Check sheet for the modelled part. Datum: model origin and axes. Units: mm. A direction names the side the tool comes from. Round coordinates to 2 decimals unless told otherwise and drop trailing zeros. Order: outer loops, then holes, each group sorted by start corner. A loop starts at its lowest first (then second) coordinate and runs counter-clockwise, first axis right, second up. Notation, with made-up numbers: M 85.25,33 L 112.25,33 A9 cw 112.25,40 Z; hole C -38.75,-36 d3. An arc over 180 degrees is marked long. One line per item, written item: value. Start each with the question number.
(1) Depth check by flat-ended pin: pin 1 Ø6 at (x, y) = (2, -2) entering from +Z. Enter the tip coordinate at first touch or a pass-through.
(2) Release check for a two-part mould opening along Z. For faces 1 (the face through (0, -11, 3)), 2 (the face through (-1, -1, 0)), 3 (the face through (-10.5, -1, 9)) record: released by +Z, released by -Z, zero draft, split by the parting line, or undercut.
(3) Cross-section at D-D, the plane x = 2. Enter the section's corners in (y, z).
(4) Cross-section at C-C, the plane z = 2. Enter the section's corners in (x, y).
(5) Thickness scan on L1, parallel to X at y = -6.75, z = 3.5; L2, parallel to Y at x = -2, z = 17.25; L3, parallel to X at y = -10.25, z = 13.25. Record the ranges inside material, lowest first.
(6) Access from +Z, -Z, +X, -X, +Y, -Y to the whole of each face (thin tool, end or side, straight path). Record for faces 4 (the face through (-2.9, -11, 9)), 5 (the face through (8.5, -1, 9)), 6 (the face through (-9, 0, 10)), 7 (the face through (6.5, 10, 11)), 8 (the face through (-2.5, 10, 12)).
(7) Cross-section at B-B, the plane x = 5.5. Enter the section's corners in (y, z).
(8) Cross-section at A-A, the plane y = -11.25. Enter the section's corners in (x, z).
Autodesk Inventor part; units mm, degrees
ref_plane "YZ Plane" through (0, 0, 0) normal (1, 0, 0) x (0, 1, 0)
ref_plane "XZ Plane" through (0, 0, 0) normal (0, 1, 0) x (-1, 0, 0)
ref_plane "XY Plane" through (0, 0, 0) normal (0, 0, 1) x (1, 0, 0)
sketch "Náčrt1" plane through (0, 0, 0) normal (0, 0, 1) x (1, 0, 0)
  line L0 (0, 18.2) -> (0, -18.2)
  line L1 (-14.7, 0) -> (14.7, 0)
  line L2 (-10.5, 13) -> (10.5, 13)
  line L3 (10.5, 13) -> (10.5, -13)
  line L4 (10.5, -13) -> (-10.5, -13)
  line L5 (-10.5, -13) -> (-10.5, 13)
  line L6 (-10.5, 13) -> (10.5, -13) construction
  line L7 (10.5, 13) -> (-10.5, -13) construction
  point P0 (0, 0)
  dimension "d0" = 21
  dimension "d1" = 26
extrude "Vysunutí1" add sketch "Náčrt1" along normal blind 18
sketch "Náčrt4" plane through (0, 0, 18) normal (0, 0, 1) x (1, 0, 0)
  line L0 (-14.7, 0) -> (14.7, 0)
  line L1 (0, 18.2) -> (0, -18.2)
  line L2 (-10.5, -13) -> (10.5, -13)
  line L3 (10.5, -13) -> (10.5, 13)
  line L4 (10.5, 13) -> (-10.5, 13)
  line L5 (-10.5, 13) -> (-10.5, -13)
  line L6 (-9, -9.5) -> (7, -9.5)
  line L7 (7, -9.5) -> (7, 9.5)
  line L8 (7, 9.5) -> (-9, 9.5)
  line L9 (-9, 9.5) -> (-9, -9.5)
  point P0 (0, 0)
  dimension "d9" = 3.5
  dimension "d34" = 16
  dimension "d35" = 1.5
  dimension "d36" = 19
extrude "Vysunutí2" cut sketch "Náčrt4" against normal blind 16.5 contours L9 L8 L1 L0 | L0 L1 L6 L9 | L1 L8 L7 L0 | L0 L7 L6 L1
sketch "Náčrt5" plane through (-10.5, 13, 0) normal (0, 1, 0) x (1, 0, 0)
  line L0 (21, 0) -> (0, 0)
  line L1 (0, 0) -> (0, -18)
  line L2 (21, -18) -> (0, -18)
  line L3 (21, 0) -> (21, -18)
  line L4 (17, -15) -> (8, -15)
  line L5 (8, -15) -> (8, -8)
  line L6 (8, -8) -> (17, -8)
  line L7 (17, -8) -> (17, -15)
  line L8 (17, -15) -> (8, -8) construction
  line L9 (8, -15) -> (17, -8) construction
  point P0 (10.5, 0)
  point P1 (12.5, -11.5)
  dimension "d12" = 9
  dimension "d13" = 7
  dimension "d14" = 3
  dimension "d15" = 8
extrude "Vysunutí3" cut sketch "Náčrt5" against normal up to surface (3.5 mm away) contours L4 L5 L6 L7
sketch "Náčrt6" plane through (-10.5, -13, 0) normal (0, -1, 0) x (1, 0, 0)
  line L0 (0, 0) -> (21, 0)
  line L1 (21, 0) -> (21, 18)
  line L2 (0, 18) -> (21, 18)
  line L3 (0, 0) -> (0, 18)
  line L4 (7.6, 15) -> (13.4, 15)
  line L5 (13.4, 15) -> (13.4, 3)
  line L6 (13.4, 3) -> (7.6, 3)
  line L7 (7.6, 3) -> (7.6, 15)
  line L8 (7.6, 15) -> (13.4, 3) construction
  line L9 (13.4, 15) -> (7.6, 3) construction
  point P0 (10.5, 0)
  point P1 (10.5, 9)
  dimension "d18" = 5.8
  dimension "d19" = 12
  dimension "d20" = 10.5
  dimension "d21" = 9
extrude "Vysunutí4" cut sketch "Náčrt6" against normal up to surface (3.5 mm away) contours L4 L5 L6 L7
sketch "Náčrt8" plane through (0, 0, 18) normal (0, 0, 1) x (1, 0, 0)
  line L0 (7, 9.5) -> (7, -9.5)
  line L1 (7, -9.5) -> (-9, -9.5)
  line L2 (-9, -9.5) -> (-9, 9.5)
  line L3 (-9, 9.5) -> (7, 9.5)
  line L4 (-10.5, -13) -> (10.5, -13)
  line L5 (10.5, -13) -> (10.5, 13)
  line L6 (10.5, 13) -> (-10.5, 13)
  line L7 (-10.5, 13) -> (-10.5, -13)
  line L8 (-10.5, 11) -> (8.5, 11)
  line L9 (8.5, -13) -> (8.5, 11)
  point P0 (0, 0)
  dimension "d37" = 1.5
  dimension "d38" = 1.5
extrude "Vysunutí6" cut sketch "Náčrt8" against normal through all contours L9 L8 L7 L6 L5 L4
properties part number "senzor_obal_3D tisk"
Values found:
1. pin 1: z = 1.5
2. face 1: undercut
2. face 2: released by -Z
2. face 3: zero draft
3. outline: M -13,0 L 11,0 L 11,8 L 9.5,8 L 9.5,1.5 L -9.5,1.5 L -9.5,3 L -13,3 Z; M -13,15 L -9.5,15 L -9.5,18 L -13,18 Z; M 9.5,15 L 11,15 L 11,18 L 9.5,18 Z
4. outline: M -10.5,-13 L 8.5,-13 L 8.5,11 L -10.5,11 Z; hole M -9,-9.5 L 7,-9.5 L 7,9.5 L -9,9.5 Z
5. L1: -10.5 to -9, 7 to 8.5
5. L2: -13 to -9.5, 9.5 to 11
5. L3: -10.5 to -2.9, 2.9 to 8.5
6. face 4: -Y
6. face 5: +Z, -Z, +X, +Y, -Y
6. face 6: +Z
6. face 7: +Y
6. face 8: +Y, -Y
7. outline: M -13,0 L 11,0 L 11,8 L 9.5,8 L 9.5,1.5 L -9.5,1.5 L -9.5,18 L -13,18 Z; M 9.5,15 L 11,15 L 11,18 L 9.5,18 Z
8. outline: M -10.5,0 L 8.5,0 L 8.5,18 L -10.5,18 Z; hole M -2.9,3 L 2.9,3 L 2.9,15 L -2.9,15 Z
